```python
from build123d import *

# Parameters (mm, degrees)
SKETCH_1_R          = 28.5
SKETCH_1_R_2        = 14
SKETCH_1_R_3        = 3
EXTRUDE_1_DEPTH     = 12
SKETCH_2_R          = 4.75
CUT_EXTRUDE_1_DEPTH = 5.4


with BuildPart() as part:
    # 草图1 → 凸台-拉伸1 (new body)
    with BuildSketch(Plane.XY):
        Circle(SKETCH_1_R)
        Circle(SKETCH_1_R_2, mode=Mode.SUBTRACT)
        with Locations((0, 22.5)):
            Circle(SKETCH_1_R_3, mode=Mode.SUBTRACT)
        with Locations((22.5, 0)):
            Circle(SKETCH_1_R_3, mode=Mode.SUBTRACT)
        with Locations((0, -22.5)):
            Circle(SKETCH_1_R_3, mode=Mode.SUBTRACT)
        with Locations((-22.5, 0)):
            Circle(SKETCH_1_R_3, mode=Mode.SUBTRACT)
    extrude(amount=EXTRUDE_1_DEPTH)

    # 草图2 → 切除-拉伸1 (cut)
    with BuildSketch(Plane.XY.offset(12)):
        with Locations((0, 22.5)):
            Circle(SKETCH_2_R)
        with Locations((22.5, 0)):
            Circle(SKETCH_2_R)
        with Locations((0, -22.5)):
            Circle(SKETCH_2_R)
        with Locations((-22.5, 0)):
            Circle(SKETCH_2_R)
    extrude(amount=-CUT_EXTRUDE_1_DEPTH, mode=Mode.SUBTRACT)


solid = part.part
```
The listing builds one solid part. Answer for the finished solid, in the listing's coordinates (mm). A direction names the side the tool comes from. Coordinates: 2 decimals unless noted, no trailing zeros. Write each loop counter-clockwise with the first axis right and the second up, starting at its lowest first coordinate (ties: lowest second). Pieces come first, ordered by that corner, then holes.
Q1. Section D-D, the plane x = -22.5 is taken. Write down the section's boundary in (y, z), then the cut area to 3 significant figures.
Returned:
outline: (-17.49, 0) - (-3, 0) - (-3, 6.6) - (-4.75, 6.6) - (-4.75, 12) - (-17.49, 12) - close; (3, 0) - (17.49, 0) - (17.49, 12) - (4.75, 12) - (4.75, 6.6) - (3, 6.6) - close
area: 329 mm2
Q2. Section C-C, the plane z = 10 is taken. Write down the section's boundary in (x, y), then the cut area to 3 significant figures.
Returned:
outline: circle Ø57 at (0, 0); hole circle Ø9.5 at (-22.5, 0); hole circle Ø28 at (0, 0); hole circle Ø9.5 at (0, -22.5); hole circle Ø9.5 at (0, 22.5); hole circle Ø9.5 at (22.5, 0)
area: 1,650 mm2
Q3. Given P1, Ø6, axis at x = -19.5, z = 5, coming from the -Y side; P2, Ø5, axis at x = 12.5, z = 10.5, coming from the -Y side; P3, Ø8.5, axis at x = -22.5, y = 0, coming from the +Z side, each flat-ended and moving along its own axis, determine where each tip first touches the part or whether it passes through.
Returned:
P1: stops at y = -23.24
P2: stops at y = -26.69
P3: stops at z = 6.6
Q4. Find the intervals of material crossed by line 1 along Y through (x, z) = (0, 10.8); line 2 along Y through (x, z) = (-22.5, 9.2); line 3 along X through (y, z) = (-13, 8.5), in increasing order.
Returned:
line 1: y = -28.5 to -27.25, -17.75 to -14, 14 to 17.75, 27.25 to 28.5
line 2: y = -17.49 to -4.75, 4.75 to 17.49
line 3: x = -25.36 to -5.2, 5.2 to 25.36
Q5. The mould has two halves that part along X. Classify faces 3 (the flat face through (-13, 7, 0)), 4 (the cylindrical face through (-18.112, -1.819, 9.338)), 5 (the cylindrical face through (26.327, -10.916, 5.916)): released by +X, released by -X, zero draft, split by the parting line, or undercut.
Returned:
face 3: zero draft
face 4: undercut
face 5: split by the parting line
Q6. Which of the six approach directions +Z, -Z, +X, -X, +Y, -Y give full straight-line access (tool end or side, diameter ignored) to faces 1 (the cylindrical face through (27.03, 1.43, 9.34)), 2 (the cylindrical face through (-25.5, 0.1, 3.3))?
Returned:
face 1: +Z
face 2: +Z, -Z
Q7. Section A-A, the plane y = 0 is taken. Write down the section's boundary in (x, z).
Returned:
outline: (-28.5, 0) - (-25.5, 0) - (-25.5, 6.6) - (-27.25, 6.6) - (-27.25, 12) - (-28.5, 12) - close; (-19.5, 0) - (-14, 0) - (-14, 12) - (-17.75, 12) - (-17.75, 6.6) - (-19.5, 6.6) - close; (14, 0) - (19.5, 0) - (19.5, 6.6) - (17.75, 6.6) - (17.75, 12) - (14, 12) - close; (25.5, 0) - (28.5, 0) - (28.5, 12) - (27.25, 12) - (27.25, 6.6) - (25.5, 6.6) - close
